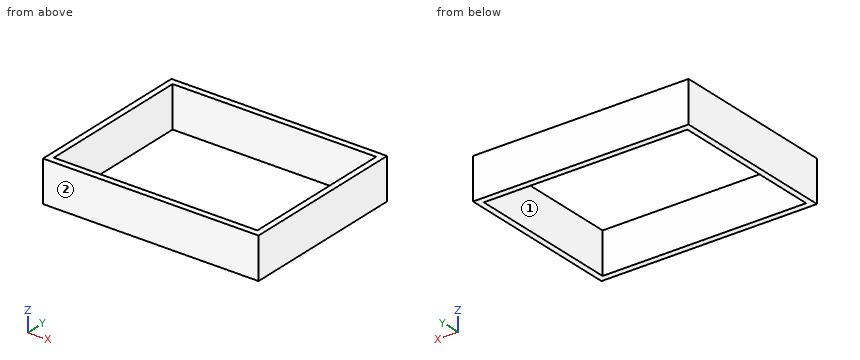
```python
from build123d import *

# Parameters (mm, degrees)
F0_W     = 133.195832
F0_H     = 104.52173
F1_DEPTH = 25.4


with BuildPart() as f1:
    # F0 (on Top) → F1 (new body)
    with BuildSketch(Plane.XY):
        Rectangle(F0_W, F0_H)
        Polygon((-62.898032, -7.168526), (-62.898032, 48.329741), (-37.461329, 48.329741), (-34.455173, 48.329741), (2.312429, 48.329741), (62.898032, 48.329741), (62.898032, 26.824163), (62.898032, -48.329741), (-62.898032, -48.329741), (-62.898032, -9.24971), align=None, mode=Mode.SUBTRACT)
    extrude(amount=F1_DEPTH)


solid = f1.part
```
Could you check a few things on this model? Use its own coordinates, in mm. Face numbers are marked on the shaded views. A direction names the side the tool comes from. Coordinates: 2 decimals unless noted, no trailing zeros. Order: outer loops, then holes, each group sorted by start corner. A loop starts at its lowest first (then second) coordinate and runs counter-clockwise, first axis right, second up. Notation, with made-up numbers: M 53.5,46.5 L 108.5,46.5 A33 cw 108.5,75.5 Z; hole C 7,88 d2. An arc over 180 degrees is marked long. Use a Markdown table: item, result. Add a question column.
Q1. I want a section at C-C on z = 12.5. List the corners of the cut face in (x, y) for me, then the cut area to 3 significant figures.
Q2. If I drill on L1, parallel to Y at x = -39, z = 15.5; L2, parallel to X at y = 5.5, z = 19.75, over which ranges is the centre line in solid material (lowest first)?
Q3. I want a section at A-A on y = 33. List the corners of the cut face in (x, z) for me.
Q4. I want a section at B-B on x = 20. List the corners of the cut face in (y, z) for me.
Q5. Which directions (+Z, -Z, +X, -X, +Y, -Y) give clear straight access to the entire face, cutting with the end or side of a thin tool? Please do the marked faces 1 and 2.
Checked values:
| question | item | result |
|---|---|---|
| 1 | outline | M -66.6,-52.26 L 66.6,-52.26 L 66.6,52.26 L -66.6,52.26 Z; hole M -62.9,-48.33 L 62.9,-48.33 L 62.9,48.33 L -62.9,48.33 Z |
| 1 | area | 1,760 mm² |
| 2 | L1 | -52.26 to -48.33, 48.33 to 52.26 |
| 2 | L2 | -66.6 to -62.9, 62.9 to 66.6 |
| 3 | outline | M -66.6,0 L -62.9,0 L -62.9,25.4 L -66.6,25.4 Z; M 62.9,0 L 66.6,0 L 66.6,25.4 L 62.9,25.4 Z |
| 4 | outline | M -52.26,0 L -48.33,0 L -48.33,25.4 L -52.26,25.4 Z; M 48.33,0 L 52.26,0 L 52.26,25.4 L 48.33,25.4 Z |
| 5 | face 1 | +Z, -Z |
| 5 | face 2 | +Z, -Z, +X, -X, -Y |
